Geometry check sheet. Reference: the model listing, model coordinates, mm. Face numbers are marked on the shaded views. A direction names the side the tool comes from. Round coordinates to 2 decimals unless told otherwise and drop trailing zeros. Order: outer loops, then holes, each group sorted by start corner. A loop starts at its lowest first (then second) coordinate and runs counter-clockwise, first axis right, second up. Notation, with made-up numbers: (28, 88) -> (58, 88) arc R32 cw to (58, 125) -> close; hole circle Ø11 at (81, -14). An arc over 180 degrees is marked (long way). Use a Markdown table: item, result. Add a question column.
Item 1: Set-up check for the marked faces 5, 6 and 7: record each of +Z, -Z, +X, -X, +Y, -Y from which the full face is reachable in a straight line by a thin tool's end or side.
Item 2: Mould release check, pull along Z, two halves, no side actions. Record for the marked faces 1, 2, 3 and 4: pulls with the +Z half, pulls with the -Z half, needs draft (parallel to the pull), parting line crosses it, or undercut.
Item 3: Sectioned sample at A-A, the plane y = 2. Record the cut outline in (x, z), and give its area (3 significant figures).
Item 4: Sectioned sample at B-B, the plane x = -7.5. Record the cut outline in (y, z), and give its area (3 significant figures).
Item 5: Sectioned sample at C-C, the plane z = -17. Record the cut outline in (x, y).
Item 6: Material ranges on probe 1 along Y at (x, z) = (-10.25, -15); probe 2 along X at (y, z) = (6.25, -16.75); probe 3 along Z at (x, y) = (-10, 5.5), recorded low to high. Write a range as [from, to].
Item 7: Gauge pin test, flat ends, axial feed: pin 1 Ø2.5 at (x, y) = (-10.5, 4) entering from -Z; pin 2 Ø3 at (x, y) = (-14, 3.5) entering from +Z; pin 3 Ø0.8 at (y, z) = (9.5, -16.5) entering from -X. Record the tip position at first contact, or that the pin passes through.
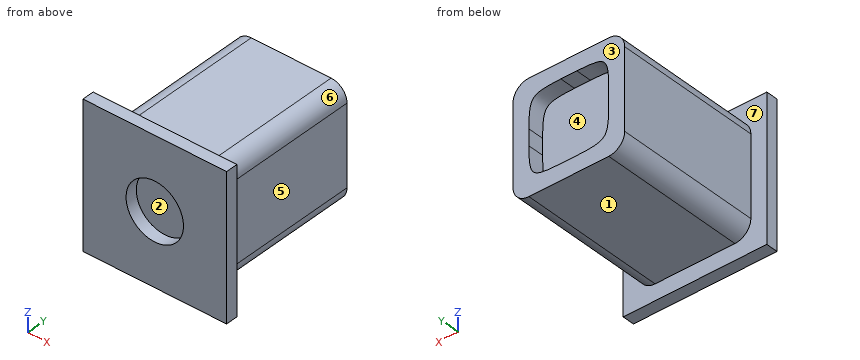
from build123d import *

# Parameters (mm, degrees)
SKETCH1_W           = 7
SKETCH1_H           = 7
SKETCH1_R           = 1.8
BOSS_EXTRUDE1_DEPTH = 10
SKETCH1_4_R         = 1.8
CUT_EXTRUDE1_DEPTH  = 0.75
SKETCH2_W           = 8
SKETCH2_H           = 0.75
BOSS_EXTRUDE2_DEPTH = 1
CIRPATTERN1_DEPTH   = 0.75
SKETCH4_W           = 5
SKETCH4_H           = 5
CUT_EXTRUDE2_DEPTH  = 1
FILLET1_SIZE        = 2
FILLET2_R           = 1


with BuildPart() as part:
    # Sketch1 → Boss-Extrude1 (new body)
    # profile 1 of 2: a face of its own
    with BuildSketch(Plane(origin=(0, 0, 0), x_dir=(1, 0, 0), z_dir=(0, 1, 0))):
        with Locations((-10.213000206, 16.666176773)):
            Rectangle(SKETCH1_W, SKETCH1_H)
        with Locations((-10.213000206, 16.666176773)):
            Circle(SKETCH1_R, mode=Mode.SUBTRACT)
    # profile 2 of 2: a face of its own
    with BuildSketch(Plane(origin=(0, 0, 0), x_dir=(1, 0, 0), z_dir=(0, 1, 0))):
        with Locations((-10.213000206, 16.666176773)):
            Circle(SKETCH1_R)
    extrude(amount=BOSS_EXTRUDE1_DEPTH)

    # Sketch1<4> → Cut-Extrude1 (cut)
    with BuildSketch(Plane(origin=(0, 0, 0), x_dir=(1, 0, 0), z_dir=(0, 1, 0))):
        with Locations(Location((-10.213000206, 16.666176773, 0), (0, 0, 270))):
            Circle(SKETCH1_4_R)
    extrude(amount=CUT_EXTRUDE1_DEPTH, mode=Mode.SUBTRACT)

    # Sketch2 → Boss-Extrude2 (add)
    with BuildSketch(Plane(origin=(-6.713000206, 0, 0), x_dir=(0, 0, -1), z_dir=(1, 0, 0))):
        with Locations((17.166176773, 0.375)):
            Rectangle(SKETCH2_W, SKETCH2_H)
    extrude(amount=BOSS_EXTRUDE2_DEPTH)

    # CirPattern1: read off the stored shape, not the designer's step
    # CirPattern1 outline → CirPattern1 (add)
    with BuildSketch(Plane(origin=(0, 0, 0), x_dir=(1, 0, 0), z_dir=(0, 1, 0))):
        Polygon((-6.713000206, 21.166176773), (-14.713000206, 21.166176773), (-14.713000206, 12.166176773), (-5.713000206, 12.166176773), (-5.713000206, 13.166176773), (-13.713000206, 13.166176773), (-13.713000206, 20.166176773), (-6.713000206, 20.166176773), align=None)
    extrude(amount=CIRPATTERN1_DEPTH)

    # Sketch4 → Cut-Extrude2 (cut)
    with BuildSketch(Plane(origin=(0, 10, 0), x_dir=(1, 0, 0), z_dir=(0, 1, 0))):
        with Locations((-10.213000206, 16.666176773)):
            Rectangle(SKETCH4_W, SKETCH4_H)
    extrude(amount=-CUT_EXTRUDE2_DEPTH, mode=Mode.SUBTRACT)

    # Fillet1
    # a fillet whose section is not a circle: 2 mm, written as the material it adds along each edge
    with BuildSketch(Plane(origin=(-12.713000206, 10, -19.166176773), x_dir=(0, 0, 1), z_dir=(0, -1, 0)), Plane(origin=(-7.713000206, 10, -19.166176773), x_dir=(-1, 0, 0), z_dir=(0, -1, 0)), Plane(origin=(-12.713000206, 10, -14.166176773), x_dir=(1, 0, 0), z_dir=(0, -1, 0))) as fillet1_piece_1:
        with BuildLine():
            Bezier((FILLET1_SIZE, 0), (0, 0), (0, -FILLET1_SIZE), weights=[1, 2.333333333, 1])
            Line((0, -FILLET1_SIZE), (0, 0))
            Line((0, 0), (FILLET1_SIZE, 0))
        make_face()
    extrude(amount=6)
    with BuildSketch(Plane(origin=(-7.713000206, 10, -14.166176773), x_dir=(-1, 0, 0), z_dir=(0, -1, 0))) as fillet1_piece_2:
        with BuildLine():
            Bezier((FILLET1_SIZE, 0), (0, 0), (0, FILLET1_SIZE), weights=[1, 2.333333333, 1])
            Line((0, FILLET1_SIZE), (0, 0))
            Line((0, 0), (FILLET1_SIZE, 0))
        make_face()
    extrude(amount=6)

    # Fillet2
    fillet2_edges = [part.edges().sort_by_distance(p)[0] for p in [
        (-6.713000206, 5.375, -13.166176773),
        (-13.713000206, 5.375, -13.166176773),
        (-13.713000206, 5.375, -20.166176773),
        (-6.713000206, 5.375, -20.166176773),
    ]]
    fillet(fillet2_edges, radius=FILLET2_R)


solid = part.part
Found:
| question | item | result |
|---|---|---|
| 1 | face 5 | +Z, -Z, +X, +Y |
| 1 | face 6 | +Z, +X, +Y |
| 1 | face 7 | +Y |
| 2 | face 1 | pulls with the -Z half |
| 2 | face 2 | undercut |
| 2 | face 3 | needs draft |
| 2 | face 4 | undercut |
| 3 | outline | (-13.71, -19.17) arc R1 ccw to (-12.71, -20.17) -> (-7.71, -20.17) arc R1 ccw to (-6.71, -19.17) -> (-6.71, -14.17) arc R1 ccw to (-7.71, -13.17) -> (-12.71, -13.17) arc R1 ccw to (-13.71, -14.17) -> close |
| 3 | area | 48.1 mm2 |
| 4 | outline | (0, -21.17) -> (0.75, -21.17) -> (0.75, -20.14) -> (10, -20.14) -> (10, -13.19) -> (0.75, -13.19) -> (0.75, -12.17) -> (0, -12.17) -> close |
| 4 | area | 71.1 mm2 |
| 5 | outline | (-14.71, 0) -> (-11.98, 0) -> (-11.98, 0.75) -> (-8.44, 0.75) -> (-8.44, 0) -> (-5.71, 0) -> (-5.71, 0.75) -> (-6.71, 0.75) -> (-6.71, 10) -> (-7.71, 10) -> (-7.71, 9) -> (-12.71, 9) -> (-12.71, 10) -> (-13.71, 10) -> (-13.71, 0.75) -> (-14.71, 0.75) -> close |
| 6 | probe 1 | y = [0.75, 9] |
| 6 | probe 2 | x = [-13.71, -6.71] |
| 6 | probe 3 | z = [-20.17, -13.17] |
| 7 | pin 1 | stops at z = -20.17 |
| 7 | pin 2 | stops at z = -13.17 |
| 7 | pin 3 | stops at x = -13.71 |
